Input: part model. Units: mm. Frame: model coordinates. Face numbers are marked on the shaded views. Give positions to 0.01 mm unless a question says otherwise; leave off trailing zeros. Order: outer loops, then holes, each group sorted by start corner. A loop starts at its lowest first (then second) coordinate and runs counter-clockwise, first axis right, second up. Notation, with made-up numbers: (75.5, 54) - (112.5, 54) arc R17 ccw to (112.5, 58) - close; hole circle Ø7 at (-38, 23). An arc over 180 degrees is marked (long way). Answer in a Markdown table with one row per item. Add a question column.
from build123d import *

# Parameters (mm, degrees)
SKETCH1_R           = 1.9
BOSS_EXTRUDE1_DEPTH = 1.3
SKETCH2_R           = 1
BOSS_EXTRUDE2_DEPTH = 10
CHAMFER1_SIZE       = 1.1
CUT_EXTRUDE1_DEPTH  = 0.3


with BuildPart() as part:
    # Sketch1 → Boss-Extrude1 (new body)
    with BuildSketch(Plane(origin=(0, 0, 0), x_dir=(1, 0, 0), z_dir=(0, 1, 0))):
        with Locations(Location((0, 0, 0), (0, 0, 270))):
            Circle(SKETCH1_R)
    extrude(amount=BOSS_EXTRUDE1_DEPTH)

    # Sketch2 → Boss-Extrude2 (add)
    with BuildSketch(Plane.XZ):
        with Locations(Location((0, 0, 0), (0, 0, 270))):
            Circle(SKETCH2_R)
    extrude(amount=-BOSS_EXTRUDE2_DEPTH)

    # Chamfer1
    # the kernel refuses this chamfer: 1.1 mm, written as the material it takes off along each edge
    with BuildSketch(Plane(origin=(0, 1.3, 0), x_dir=(0, 0, 1), z_dir=(-1, 0, 0))) as chamfer1_piece_1_section:
        Polygon((1.9, -CHAMFER1_SIZE), (1.9 - CHAMFER1_SIZE, 0), (1.9, 0), align=None)
    chamfer1_piece_1 = revolve(axis=Axis((0, 1.3, 0), (0, 1, 0)), mode=Mode.PRIVATE)
    chamfer1_piece_1 = chamfer1_piece_1 - Plane(origin=(0, 0.647474875, 0), x_dir=(0, 0, -1), z_dir=(0, -1, 0)) * Cylinder(1, 8, mode=Mode.PRIVATE)
    add(chamfer1_piece_1, mode=Mode.SUBTRACT)

    # Sketch3 → Cut-Extrude1 (cut)
    with BuildSketch(Plane.XZ):
        Polygon((-0.25, 1.5), (-0.25, 0.25), (-1.5, 0.25), (-1.5, -0.25), (-0.25, -0.25), (-0.25, -1.5), (0.25, -1.5), (0.25, -0.25), (1.5, -0.25), (1.5, 0.25), (0.25, 0.25), (0.25, 1.5), align=None)
    extrude(amount=-CUT_EXTRUDE1_DEPTH, mode=Mode.SUBTRACT)


solid = part.part
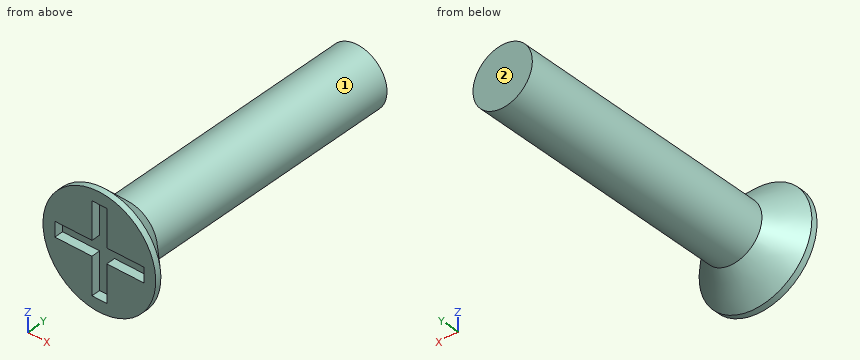
Q1. Section B-B, the plane z = 0. Return loops of the section in (x, y).
Q2. Section C-C, the plane y = 8.75. Return loops of the section in (x, z), then the cut area to 3 significant figures.
Q3. Line query: probe 1 along X at (y, z) = (9.25, 0.05); probe 2 along Y at (x, z) = (0, -0.45); probe 3 along Y at (x, z) = (-0.85, 1.45). Output: solid intervals per line, ascending.
Q4. Pull-direction query (Z, two-part tool) for the marked faces 1 and 2; classes: +Z half, -Z half, draft (parallel to the pull), parting line (faces both ways), or undercut.
Q5. Contact query for flat-ended pins moving along their axis: P1, Ø1, axis at x = 1, y = 3.5, coming from the -Z side; P2, Ø1, axis at x = -1, y = 6, coming from the +Z side. Output: stop coordinate, or through.
Q6. Section A-A, the plane x = 0. Return loops of the section in (y, z).
Computed:
| question | item | result |
|---|---|---|
| 1 | outline | (-1.9, 0) - (-1.5, 0) - (-1.5, 0.3) - (1.5, 0.3) - (1.5, 0) - (1.9, 0) - (1.9, 0.2) - (1, 1.1) - (1, 10) - (-1, 10) - (-1, 1.1) - (-1.9, 0.2) - close |
| 2 | outline | circle Ø2 at (0, 0) |
| 2 | area | 3.14 mm^2 |
| 3 | probe 1 | x = -1 to 1 |
| 3 | probe 2 | y = 0.3 to 10 |
| 3 | probe 3 | y = 0 to 0.42 |
| 4 | face 1 | parting line |
| 4 | face 2 | draft |
| 5 | P1 | stops at z = -0.87 |
| 5 | P2 | stops at z = 0.87 |
| 6 | outline | (0, -1.9) - (0.2, -1.9) - (1.1, -1) - (10, -1) - (10, 1) - (1.1, 1) - (0.2, 1.9) - (0, 1.9) - (0, 1.5) - (0.3, 1.5) - (0.3, -1.5) - (0, -1.5) - close |
